from build123d import *

# Parameters (mm, degrees)
SKETCH1_W           = 40
SKETCH1_H           = 35
SKETCH1_R           = 3.125
BOSS_EXTRUDE1_DEPTH = 5
SKETCH1_3_W         = 40
SKETCH1_3_H         = 5
BOSS_EXTRUDE2_DEPTH = 40
FILLET1_R           = 6.25
SKETCH2_R           = 2.5
CUT_EXTRUDE1_DEPTH  = 67.520673478


with BuildPart() as part:
    # Sketch1 → Boss-Extrude1 (new body)
    with BuildSketch(Plane.XY):
        with Locations((20, 22.5)):
            Rectangle(SKETCH1_W, SKETCH1_H)
        with Locations((20, 25)):
            Circle(SKETCH1_R, mode=Mode.SUBTRACT)
    extrude(amount=BOSS_EXTRUDE1_DEPTH)

    # Sketch1_3 → Boss-Extrude2 (add)
    with BuildSketch(Plane.XY):
        with Locations((20, 2.5)):
            Rectangle(SKETCH1_3_W, SKETCH1_3_H)
    extrude(amount=BOSS_EXTRUDE2_DEPTH)

    # Fillet1
    fillet1_edges = [part.edges().sort_by_distance(p)[0] for p in [
        (20, 0, 0),
    ]]
    fillet(fillet1_edges, radius=FILLET1_R)

    # Sketch2 → Cut-Extrude1 (cut, through all)
    with BuildSketch(Plane(origin=(0, 5, 0), x_dir=(1, 0, 0), z_dir=(0, 1, 0))):
        with Locations(Location((10, -22.5, 0), (0, 0, 270))):
            Circle(SKETCH2_R)
        with Locations(Location((30, -22.5, 0), (0, 0, 90))):
            Circle(SKETCH2_R)
    extrude(amount=-CUT_EXTRUDE1_DEPTH, mode=Mode.SUBTRACT)


solid = part.part
CAD build for the part. Positions are in the model's coordinates, mm. A direction names the side the tool comes from. Coordinates: 2 decimals unless noted, no trailing zeros. Loops run counter-clockwise (first coordinate to the right, second up) from the corner with the lowest first, then second, coordinate; pieces in that order, holes last. Notation, with made-up numbers: (21, -37.5) -> (66, -37.5) arc R12 cw to (66, -26.5) -> close; hole circle Ø4 at (29, -7). An arc over 180 degrees is marked (long way). One line per item, written item: value.
1. Slice it at B-B on z = 22.5. Write the cut outline in (x, y).
Answers:
outline: (0, 0) -> (7.5, 0) -> (7.5, 5) -> (0, 5) -> close; (12.5, 0) -> (27.5, 0) -> (27.5, 5) -> (12.5, 5) -> close; (32.5, 0) -> (40, 0) -> (40, 5) -> (32.5, 5) -> close
2. Which spindle directions (+Z, -Z, +X, -X, +Y, -Y) get a long thin tool onto all of the face, cutting with end or side? Do faces 1 (the face through (20, 19, 5)), 2 (the face through (0, 4, 11)). Say none if no direction does.
Answers:
face 1: +Z, +X, -X, +Y
face 2: +Z, -Z, -X, +Y, -Y
3. Slice it at A-A on x = 20. Write the cut outline in (y, z) (3 decimals).
Answers:
outline: (0, 6.25) arc R6.25 ccw to (6.25, 0) -> (21.875, 0) -> (21.875, 5) -> (5, 5) -> (5, 40) -> (0, 40) -> close; (28.125, 0) -> (40, 0) -> (40, 5) -> (28.125, 5) -> close
4. Slice it at C-C on y = 25. Write the cut outline in (x, z) (3 decimals), and give its area (3 significant figures).
Answers:
outline: (0, 0) -> (16.875, 0) -> (16.875, 5) -> (0, 5) -> close; (23.125, 0) -> (40, 0) -> (40, 5) -> (23.125, 5) -> close
area: 169 mm^2
5. Drill centre lines: line 1 (X direction, y = 2.85, z = 22.5); line 2 (X direction, y = 3, z = 22); line 3 (Y direction, x = 2.5, z = 11.5). Where is each one in solid material? Low to high. Write a range as [from, to].
Answers:
line 1: x = [0, 7.5], [12.5, 27.5], [32.5, 40]
line 2: x = [0, 7.55], [12.45, 27.55], [32.45, 40]
line 3: y = [0, 5]
6. Flat gauge pins, fed straight in: P1, Ø2, axis at x = 27, z = 19.5, coming from the +Y side; P2, Ø10, axis at x = 16, z = 27, coming from the -Y side; P3, Ø5.5, axis at x = 20, y = 25, coming from the +Z side (3 decimals). Where does each tip first touch, or does it go through?
Answers:
P1: stops at y = 5
P2: stops at y = 0
P3: passes through
7. Pull direction Y, two halves, no side cores. Call faces 3 (the face through (19.6, 28.1, 2.5)), 4 (the face through (40, 4, 11)), 5 (the face through (20, 40, 2)): pulls with the +Y half, pulls with the -Y half, needs draft (parallel to the pull), parting line crosses it, or undercut.
Answers:
face 3: undercut
face 4: needs draft
face 5: pulls with the +Y half
8. Slice it at D-D on x = 36. Write the cut outline in (y, z), and give its area (3 significant figures).
Answers:
outline: (0, 6.25) arc R6.25 ccw to (6.25, 0) -> (40, 0) -> (40, 5) -> (5, 5) -> (5, 40) -> (0, 40) -> close
area: 367 mm^2
